from build123d import *

# Parameters (mm, degrees)
SKETCH_1_W          = 33
SKETCH_1_H          = 28
SKETCH_1_R          = 2
EXTRUDE_1_DEPTH     = 25
FILLET_1_R          = 4
SKETCH_2_R          = 9.5
CUT_EXTRUDE_1_DEPTH = 42.003048667


with BuildPart() as part:
    # 草图1 → 凸台-拉伸1 (new body)
    with BuildSketch(Plane.XY):
        Rectangle(SKETCH_1_W, SKETCH_1_H)
        with Locations((12.5, -10)):
            Circle(SKETCH_1_R, mode=Mode.SUBTRACT)
        with Locations((-12.5, -10)):
            Circle(SKETCH_1_R, mode=Mode.SUBTRACT)
        with Locations((-12.5, 10)):
            Circle(SKETCH_1_R, mode=Mode.SUBTRACT)
        with Locations((12.5, 10)):
            Circle(SKETCH_1_R, mode=Mode.SUBTRACT)
    extrude(amount=EXTRUDE_1_DEPTH)

    # 圆角1
    fillet_1_edges = [part.edges().sort_by_distance(p)[0] for p in [
        (16.5, -14, 12.5),
        (-16.5, -14, 12.5),
        (-16.5, 14, 12.5),
        (16.5, 14, 12.5),
    ]]
    fillet(fillet_1_edges, radius=FILLET_1_R)

    # 草图2 → 切除-拉伸1 (cut, through all)
    with BuildSketch(Plane(origin=(0, 14, 0), x_dir=(1, 0, 0), z_dir=(0, 1, 0))):
        with Locations(Location((0, -12.5, 0), (0, 0, 180))):
            Circle(SKETCH_2_R)
    extrude(amount=-CUT_EXTRUDE_1_DEPTH, mode=Mode.SUBTRACT)


solid = part.part
CAD build for the part. Positions are in the model's coordinates, mm. Coordinates: 2 decimals unless noted, no trailing zeros. Order: outer loops, then holes, each group sorted by start corner. A loop starts at its lowest first (then second) coordinate and runs counter-clockwise, first axis right, second up.
Item 1: Band-saw the part on B-B on y = 9.25. List the corners of the cut face in (x, z), plus the area to 3 significant figures.
Check sheet entries:
outline: (-16.5, 0) - (-14.35, 0) - (-14.35, 25) - (-16.5, 25) - close; (-10.65, 0) - (10.65, 0) - (10.65, 25) - (-10.65, 25) - close; (14.35, 0) - (16.5, 0) - (16.5, 25) - (14.35, 25) - close; hole circle Ø19 at (0, 12.5)
area: 356 mm2
Item 2: Two-plate mould, pull along X, no slides. Class faces 1 (the face through (11.026, -8.648, 12.325)), 2 (the face through (15.297, -12.859, 12.675)), 3 (the face through (-15.359, -12.797, 12.675)), 4 (the face through (0, 0, 0)): +X half, -X half, draft (parallel to the pull), parting line (faces both ways), or undercut.
Check sheet entries:
face 1: undercut
face 2: +X half
face 3: -X half
face 4: draft
Item 3: Band-saw the part on A-A on z = 12.5. List the corners of the cut face in (x, y), plus the area to 3 significant figures.
Check sheet entries:
outline: (-16.5, -10) arc R4 ccw to (-12.5, -14) - (-9.5, -14) - (-9.5, 14) - (-12.5, 14) arc R4 ccw to (-16.5, 10) - close; (9.5, -14) - (12.5, -14) arc R4 ccw to (16.5, -10) - (16.5, 10) arc R4 ccw to (12.5, 14) - (9.5, 14) - close; hole circle Ø4 at (-12.5, -10); hole circle Ø4 at (-12.5, 10); hole circle Ø4 at (12.5, -10); hole circle Ø4 at (12.5, 10)
area: 328 mm2
Item 4: Band-saw the part on C-C on x = 0. List the corners of the cut face in (y, z).
Check sheet entries:
outline: (-14, 0) - (14, 0) - (14, 3) - (-14, 3) - close; (-14, 22) - (14, 22) - (14, 25) - (-14, 25) - close
Item 5: Band-saw the part on D-D on y = -2.75. List the corners of the cut face in (x, z), plus the area to 3 significant figures.
Check sheet entries:
outline: (-16.5, 0) - (16.5, 0) - (16.5, 25) - (-16.5, 25) - close; hole circle Ø19 at (0, 12.5)
area: 541 mm2
Item 6: Drill centre lines: L1, parallel to Y at x = 12.5, z = 18.5; L2, parallel to X at y = 9.5, z = 3.75; L3, parallel to Y at x = -14, z = 22. Where is each one in solid material? Low to high.
Check sheet entries:
L1: y = -14 to -12, -8 to 8, 12 to 14
L2: x = -16.5 to -14.44, -10.56 to -3.7, 3.7 to 10.56, 14.44 to 16.5
L3: y = -13.71 to -11.32, -8.68 to 8.68, 11.32 to 13.71
